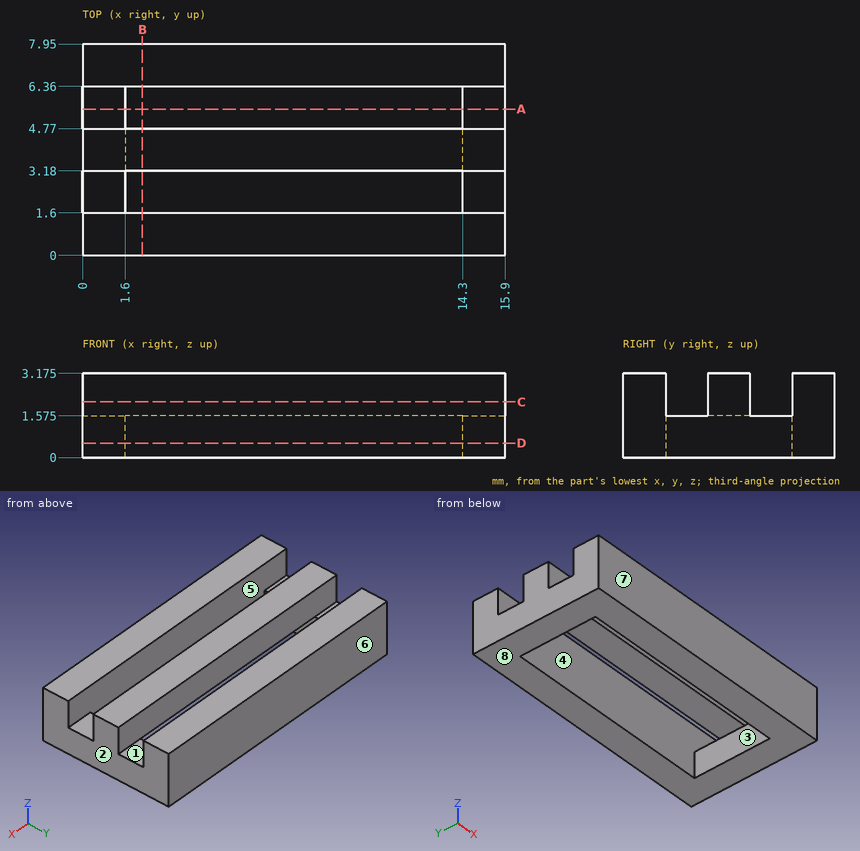
Job drawing, mm, ordinate dimensions from the low corner. One solid piece. A direction names the side the tool comes from. Give positions to 0.01 mm unless a question says otherwise; leave off trailing zeros. Write each loop counter-clockwise with the first axis right and the second up, starting at its lowest first coordinate (ties: lowest second). Pieces come first, ordered by that corner, then holes. Notation, with made-up numbers: M -32.75,62.25 L 13.25,62.25 A25 cw 13.25,74.25 Z; hole C 66,25.25 d8. An arc over 180 degrees is marked long. Put each result on its own line as item: value. Start each with the question number.
(1) Probe L1, parallel to Y at x = 6, z = 2.95; L2, parallel to Y at x = 11.75, z = 1.3; L3, parallel to X at y = 6, z = 1.35. List the from-to ranges inside material, lowest first.
(2) Band-saw the part on C-C, the plane z = 2.1. Write the cut outline in (x, y).
(3) Band-saw the part on A-A, the plane y = 5.5. Write the cut outline in (x, z) (1 decimal).
(4) Which spindle directions (+Z, -Z, +X, -X, +Y, -Y) get a long thin tool onto all of the face, cutting with end or side? Do the marked faces 1, 2, 3 and 4. Say none if no direction does.
(5) Band-saw the part on B-B, the plane x = 2.25. Give the number of separate pieces and of enclosed holes in the cut face, and give its area (3 significant figures).
(6) Flat gauge pins, fed straight in: pin 1 Ø1.7 at (x, y) = (15.5, 2.5) entering from +Z (3 decimals); pin 2 Ø0.8 at (x, y) = (15, 5.5) entering from +Z (1 decimal); pin 3 Ø1 at (x, y) = (13, 3.5) entering from -Z (1 decimal). Where does each tip first touch, or does it go through?
(7) Band-saw the part on D-D, the plane z = 0.55. Write the cut outline in (x, y).
(8) Mould opens along Y. For the marked faces 5, 6, 7 and 8 say: +Y half, -Y half, draft (parallel to the pull), parting line (faces both ways), or undercut.
Response values:
1. L1: y = 0 to 1.6, 3.18 to 4.77, 6.36 to 7.95
1. L2: y = 0 to 1.6, 6.36 to 7.95
1. L3: x = 0 to 1.6, 14.3 to 15.9
2. outline: M 0,0 L 15.9,0 L 15.9,1.6 L 0,1.6 Z; M 0,3.18 L 15.9,3.18 L 15.9,4.77 L 0,4.77 Z; M 0,6.36 L 15.9,6.36 L 15.9,7.95 L 0,7.95 Z
3. outline: M 0,0 L 1.6,0 L 1.6,1.6 L 0,1.6 Z; M 14.3,0 L 15.9,0 L 15.9,1.6 L 14.3,1.6 Z
4. face 1: +Z, +X, -X
4. face 2: +Z, -Z, +X, +Y, -Y
4. face 3: -Z
4. face 4: +Z
5. separate pieces: 3
5. enclosed holes: 0
5. area: 12.7 mm2
6. pin 1: stops at z = 3.175
6. pin 2: stops at z = 1.6
6. pin 3: stops at z = 1.6
7. outline: M 0,0 L 15.9,0 L 15.9,7.95 L 0,7.95 Z; hole M 1.6,1.6 L 14.3,1.6 L 14.3,6.36 L 1.6,6.36 Z
8. face 5: undercut
8. face 6: +Y half
8. face 7: -Y half
8. face 8: draft
